Source: CAD feature listing. Evaluate the final solid. Frame: model axes, mm. Round coordinates to 2 decimals unless told otherwise and drop trailing zeros. Loops run counter-clockwise (first coordinate to the right, second up) from the corner with the lowest first, then second, coordinate; pieces in that order, holes last. Notation, with made-up numbers: (8.5, 25.5) -> (19.5, 25.5) arc R8 ccw to (19.5, 31.5) -> close; hole circle Ø2 at (48, 15). An arc over 180 degrees is marked (long way). Write item = value, one per line.
from build123d import *

# Parameters (mm, degrees)
SKETCH1_R           = 1.47
BOSS_EXTRUDE1_DEPTH = 1.5875
SKETCH3_W           = 10.5
SKETCH3_H           = 12
CUT_EXTRUDE1_DEPTH  = 91.1946818


with BuildPart() as part:
    # Sketch1 → Boss-Extrude1 (new, symmetric)
    with BuildSketch(Plane.XY):
        Polygon((-12.5, 50), (-71.825, 50), (-71.825, 12.5), (-75, 12.5), (-75, -12.5), (-71.825, -12.5), (-71.825, -50), (-12.5, -50), (-12.5, -46.825), (-1.47, -46.825), (-1.47, -43.125), (-3.25, -43.125), (-3.25, -40.525), (-1.47, -40.525), (-1.47, -36.825), (1.47, -36.825), (1.47, -40.525), (3.25, -40.525), (3.25, -43.125), (1.47, -43.125), (1.47, -46.825), (12.5, -46.825), (12.5, -50), (71.825, -50), (71.825, -12.5), (75, -12.5), (75, 12.5), (71.825, 12.5), (71.825, 50), (12.5, 50), (12.5, 46.825), (1.47, 46.825), (1.47, 43.125), (3.25, 43.125), (3.25, 40.525), (1.47, 40.525), (1.47, 36.825), (-1.47, 36.825), (-1.47, 40.525), (-3.25, 40.525), (-3.25, 43.125), (-1.47, 43.125), (-1.47, 46.825), (-12.5, 46.825), align=None)
        with Locations((-73.4125, 0)):
            Circle(SKETCH1_R, mode=Mode.SUBTRACT)
        with Locations(Location((73.4125, 0, 0), (0, 0, 180))):
            Circle(SKETCH1_R, mode=Mode.SUBTRACT)
    extrude(amount=BOSS_EXTRUDE1_DEPTH, both=True)

    # Sketch3 → Cut-Extrude1 (cut, through all)
    with BuildSketch(Plane(origin=(0, 0, -1.5875), x_dir=(-1, 0, 0), z_dir=(0, 0, -1))):
        with Locations((-52.275, 13.144805742)):
            Rectangle(SKETCH3_W, SKETCH3_H)
    extrude(amount=-CUT_EXTRUDE1_DEPTH, mode=Mode.SUBTRACT)


solid = part.part
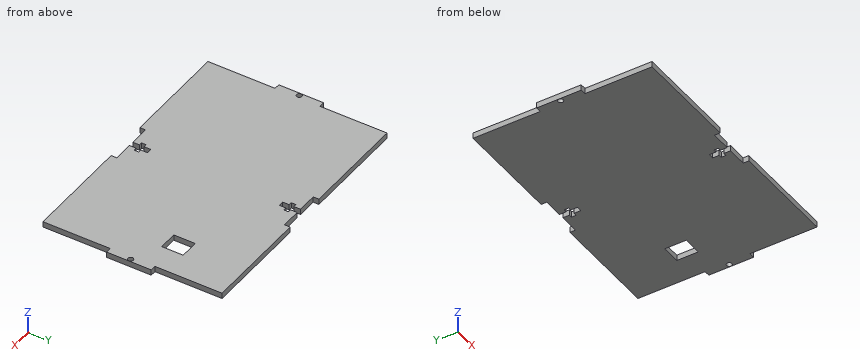
1. Contact query for flat-ended pins moving along their axis: pin 1 Ø0.5 at (x, z) = (-2, 0) entering from -Y (3 decimals); pin 2 Ø1.3 at (y, z) = (41.5, 0) entering from -X (3 decimals); pin 3 Ø1.6 at (y, z) = (-38, 0.5) entering from +X (3 decimals). Output: stop coordinate, or through.
Evaluation:
pin_1 = -46.825
pin_2 = -71.825
pin_3 = 71.825
2. Section query B-B (x = -10.5). Return the cut outline in (y, z) (1 decimal), then the cut area to 3 significant figures.
Evaluation:
outline = (-46.8, -1.6) -> (46.8, -1.6) -> (46.8, 1.6) -> (-46.8, 1.6) -> close
area = 297 mm²
3. Section query C-C (z = 0). Give the number of separate pieces and of enclosed holes in the cut face, then the cut area to 3 significant figures.
Evaluation:
separate_pieces = 1
enclosed_holes = 3
area = 14,100 mm²
4. Line query: probe 1 along Y at (x, z) = (-2.5, 1.15) (3 decimals); probe 2 along X at (y, z) = (-37.5, -1.5) (3 decimals); probe 3 along X at (y, z) = (-42, -0.3) (3 decimals). Output: solid intervals per line, ascending. Write a range as from..to.
Evaluation:
probe_1 = -46.825..-43.125, -40.525..40.525, 43.125..46.825
probe_2 = -71.825..-1.47, 1.47..71.825
probe_3 = -71.825..-3.25, 3.25..71.825
5. Section query A-A (y = 0). Return the cut outline in (x, z).
Evaluation:
outline = (-75, -1.59) -> (-74.88, -1.59) -> (-74.88, 1.59) -> (-75, 1.59) -> close; (-71.94, -1.59) -> (71.94, -1.59) -> (71.94, 1.59) -> (-71.94, 1.59) -> close; (74.88, -1.59) -> (75, -1.59) -> (75, 1.59) -> (74.88, 1.59) -> close
6. Section query D-D (y = 28.5). Return the cut outline in (x, z) (1 decimal), then the cut area to 3 significant figures.
Evaluation:
outline = (-71.8, -1.6) -> (71.8, -1.6) -> (71.8, 1.6) -> (-71.8, 1.6) -> close
area = 456 mm²
